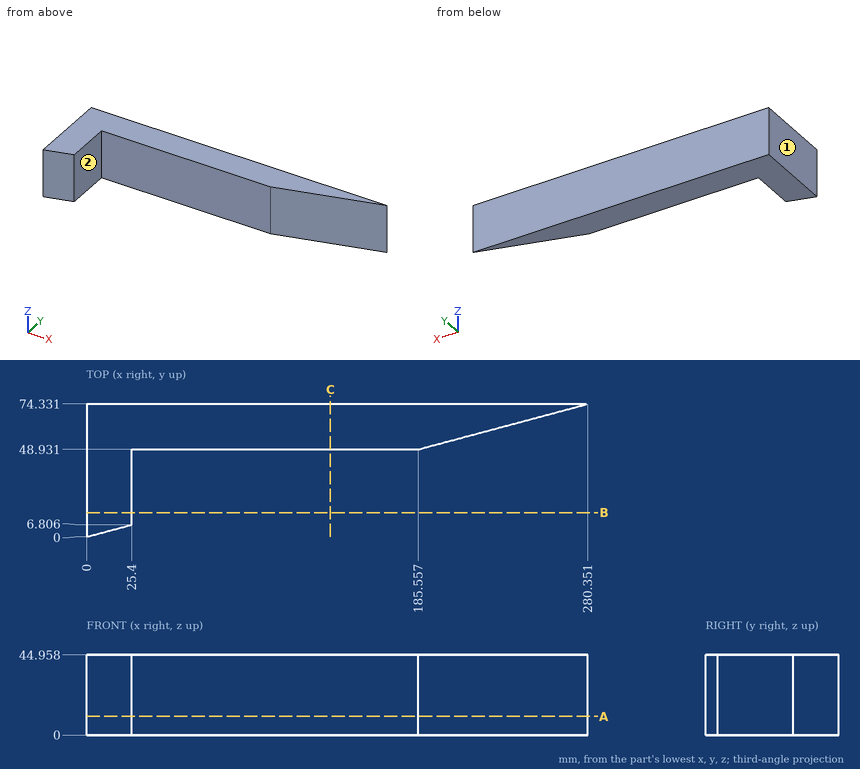
Verification items for this drawing (mm, ordinates from the low corner). A direction names the side the tool comes from. Give positions to 0.01 mm unless a question says otherwise; leave off trailing zeros. Write each loop counter-clockwise with the first axis right and the second up, starting at its lowest first coordinate (ties: lowest second). Pieces come first, ordered by that corner, then holes. Notation, with made-up numbers: (15.25, -26.5) -> (29.25, -26.5) arc R30 cw to (29.25, 6.5) -> close; hole circle Ø10 at (0, -36.75). An arc over 180 degrees is marked (long way). Use CSV: the item, a comma, the result in double quotes.
(1) Go/stop test with a flat-tipped pin: pin 1 (12.5 mm diameter, centred on y = 37.5, z = 13.5, fed in from +X). Record where the tip stops, or that it passes through.
Derived:
pin 1,"stops at x = 25.4"
(2) Sectioned sample at C-C (x = 136.5). Record the cut outline in (y, z), plus the area to 3 significant figures.
Derived:
outline,"(48.93, 0) -> (74.33, 0) -> (74.33, 44.96) -> (48.93, 44.96) -> close"
area,"1,140 mm^2"
(3) Set-up check for the marked faces 1 and 2: record each of +Z, -Z, +X, -X, +Y, -Y from which the full face is reachable in a straight line by a thin tool's end or side.
Derived:
face 1,"+Z, -Z, -X, +Y, -Y"
face 2,"+Z, -Z, +X, -Y"
(4) Material ranges on L1, parallel to Y at x = 34.5, z = 32; L2, parallel to X at y = 36.5, z = 40; L3, parallel to Y at x = 198.5, z = 24.5, recorded low to high.
Derived:
L1,"y = 48.93 to 74.33"
L2,"x = 0 to 25.4"
L3,"y = 52.4 to 74.33"
(5) Sectioned sample at A-A (z = 10.5). Record the cut outline in (x, y).
Derived:
outline,"(0, 0) -> (25.4, 6.81) -> (25.4, 48.93) -> (185.56, 48.93) -> (280.35, 74.33) -> (0, 74.33) -> close"
(6) Sectioned sample at B-B (y = 13.5). Record the cut outline in (x, z).
Derived:
outline,"(0, 0) -> (25.4, 0) -> (25.4, 44.96) -> (0, 44.96) -> close"
